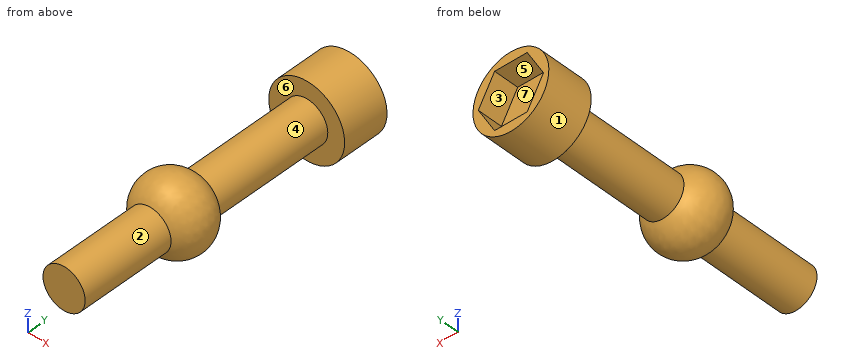
```python
from build123d import *

# Parameters (mm, degrees)
SKETCH1_R           = 1.25
BOSS_EXTRUDE1_DEPTH = 18.5
SKETCH2_R           = 2.25
BOSS_EXTRUDE2_DEPTH = 2.75
CUT_EXTRUDE1_DEPTH  = 1.5


with BuildPart() as part:
    # Sketch1 → Boss-Extrude1 (new body)
    with BuildSketch(Plane(origin=(0, 0, 0), x_dir=(1, 0, 0), z_dir=(0, 1, 0))):
        with Locations(Location((0, 0, 0), (0, 0, 270))):
            Circle(SKETCH1_R)
    extrude(amount=BOSS_EXTRUDE1_DEPTH)

    # Sketch2 → Boss-Extrude2 (add)
    with BuildSketch(Plane(origin=(0, 18.5, 0), x_dir=(1, 0, 0), z_dir=(0, 1, 0))):
        with Locations(Location((0, 0, 0), (0, 0, 270))):
            Circle(SKETCH2_R)
    extrude(amount=-BOSS_EXTRUDE2_DEPTH)

    # Sketch4 → Revolve1 (revolve)
    with BuildSketch(Plane.XY, mode=Mode.PRIVATE) as revolve1_sk:
        with BuildLine():
            Line((1.25, 8.636562631), (1.25, 5.576897201))
            ThreePointArc((1.25, 5.576897201), (2.168320153, 7.106729916), (1.25, 8.636562631))
        make_face()
    revolve(revolve1_sk.sketch.rotate(Axis((0, 0, 0), (0, 1, 0)), 90), axis=Axis((0, 0, 0), (0, 1, 0)))

    # Sketch5 → Cut-Extrude1 (cut)
    with BuildSketch(Plane(origin=(0, 18.5, 0), x_dir=(1, 0, 0), z_dir=(0, 1, 0))):
        Polygon((0.966659902, 1.674304064), (-0.966659902, 1.674304064), (-1.933319804, 0), (-0.966659902, -1.674304064), (0.966659902, -1.674304064), (1.933319804, 0), align=None)
    extrude(amount=-CUT_EXTRUDE1_DEPTH, mode=Mode.SUBTRACT)


solid = part.part
```
For this review, take the finished solid that the model builds, in its own axes (mm). Face numbers are marked on the shaded views. A direction names the side the tool comes from. Coordinates: 2 decimals unless noted, no trailing zeros. Order: outer loops, then holes, each group sorted by start corner. A loop starts at its lowest first (then second) coordinate and runs counter-clockwise, first axis right, second up. Notation, with made-up numbers: (35.25, 43) -> (55.25, 43) arc R10 ccw to (55.25, 47) -> close; hole circle Ø5 at (81.25, 18). An arc over 180 degrees is marked (long way). Answer as CSV lines item,"result".
Q1. Clearance check with flat-ended pins moving along their axes: pin 1 Ø1 at (x, z) = (0, -0.5) entering from +Y; pin 2 Ø1.5 at (y, z) = (14.5, -1) entering from +X; pin 3 Ø2 at (y, z) = (7.5, 0) entering from -X. State where each tip first meets the part, or that it passes through.
Model answer:
pin 1,"stops at y = 17"
pin 2,"stops at x = 1.22"
pin 3,"stops at x = -2.17"
Q2. For the marked faces 1, 2, 3 and 4, list the 3-axis set-ups (+Z, -Z, +X, -X, +Y, -Y) from which the entire face can be reached by the end or side of a thin tool; tool diameter is ignored.
Model answer:
face 1,"+Y, -Y"
face 2,"-Y"
face 3,"+Y"
face 4,"none"
Q3. Draft analysis for pull direction Y (two halves, no side actions). For the marked faces 5, 6 and 7, state which applies: released by +Y, released by -Y, zero draft, split by the parting line, or undercut.
Model answer:
face 5,"zero draft"
face 6,"undercut"
face 7,"released by +Y"
Q4. Wall thickness on line 1 along Y through (x, z) = (1.9, -1.1); line 2 along Y through (x, z) = (-0.15, -0.95); line 3 along X through (y, z) = (17.5, 0.2): over which ranges is each line inside the solid? List them lowest first. Write a range as [from, to].
Model answer:
line 1,"y = [15.75, 18.5]"
line 2,"y = [0, 17]"
line 3,"x = [-2.24, -1.82], [1.82, 2.24]"
Q5. We need section A-A (y = 13.5). State the section outline as (x, z) points, plus the area to 3 significant figures.
Model answer:
outline,"circle Ø2.5 at (0, 0)"
area,"4.91 mm2"
